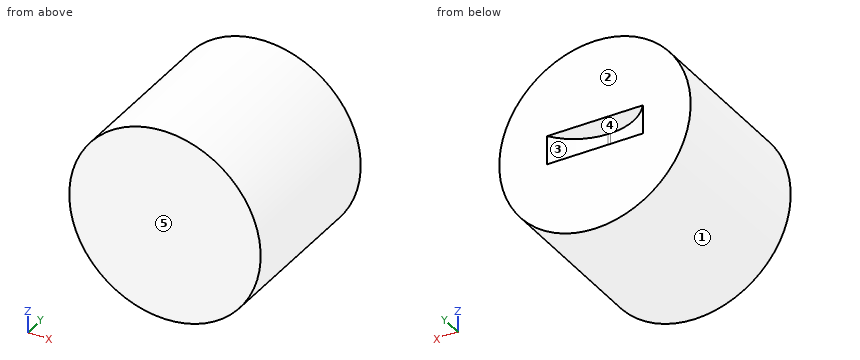
from build123d import *

# Parameters (mm, degrees)
SKETCH1_R           = 20
BOSS_EXTRUDE1_DEPTH = 35
SKETCH2_W           = 20
SKETCH2_H           = 6
CUT_EXTRUDE1_DEPTH  = 5
FILLET1_R           = 12


with BuildPart() as part:
    # Sketch1 → Boss-Extrude1 (new body)
    with BuildSketch(Plane(origin=(0, 0, 0), x_dir=(1, 0, 0), z_dir=(0, 1, 0))):
        with Locations(Location((0, 0, 0), (0, 0, 270))):
            Circle(SKETCH1_R)
    extrude(amount=BOSS_EXTRUDE1_DEPTH)

    # Sketch2 → Cut-Extrude1 (cut)
    with BuildSketch(Plane(origin=(0, 35, 0), x_dir=(1, 0, 0), z_dir=(0, 1, 0))):
        Rectangle(SKETCH2_W, SKETCH2_H)
    extrude(amount=-CUT_EXTRUDE1_DEPTH, mode=Mode.SUBTRACT)

    # Fillet1
    # the kernel refuses this fillet: 12 mm, written as the material it adds along each edge
    with BuildSketch(Plane(origin=(10, 30, 3), x_dir=(0, 1, 0), z_dir=(0, 0, -1)), Plane(origin=(-10, 30, -3), x_dir=(0, 1, 0), z_dir=(0, 0, 1))) as fillet1_piece_1:
        with BuildLine():
            CenterArc((12, -9.746794345), FILLET1_R, 125.685334713, 54.314665287)
            Line((0, -9.746794345), (0, 0))
            Line((0, 0), (5, 0))
        make_face()
    extrude(amount=6)


solid = part.part
Read the model definition and answer for the solid it produces. Units are mm, in the model's axes. Face numbers are marked on the shaded views. A direction names the side the tool comes from. Give positions to 0.01 mm unless a question says otherwise; leave off trailing zeros. Loops run counter-clockwise (first coordinate to the right, second up) from the corner with the lowest first, then second, coordinate; pieces in that order, holes last. Notation, with made-up numbers: (53, -24) - (95, -24) arc R20 cw to (95, 0) - close; hole circle Ø11 at (-40, 75.5). An arc over 180 degrees is marked (long way). Answer as CSV lines item,"result". Start each with the question number.
1) Find section A-A (z = 0). Write down the section's boundary in (x, y), then the cut area to 3 significant figures.
2) Each of these flat-tipped pins is pushed along its axis until it touches: pin 1 Ø2.5 at (x, y) = (4, 33) entering from -Z; pin 2 Ø6 at (y, z) = (16.5, 12) entering from -X; pin 3 Ø5 at (y, z) = (25, 14) entering from +X. Where does it stop, or does it pass through?
3) Determine the mould class of the marked faces 1, 2 and 3 for opening direction Z: released by +Z, released by -Z, zero draft, split by the parting line, or undercut.
4) Which of the six approach directions +Z, -Z, +X, -X, +Y, -Y give full straight-line access (tool end or side, diameter ignored) to the marked faces 4 and 5?
5) Straight lines are drawn through the part: L1, parallel to Z at x = 9.5, y = 16; L2, parallel to Z at x = -5, y = 15; L3, parallel to X at y = 25, z = 15. For each, find the intervals that lie inside material, in ascending order. Write a range as from..to.
6) Find section B-B (y = 27). Write down the section's boundary in (x, z), then the cut area to 3 significant figures.
7) Find section D-D (z = -4.5). Write down the section's boundary in (x, y), then the cut area to 3 significant figures.
8) Find section C-C (x = 17). Write down the section's boundary in (y, z), then the cut area to 3 significant figures.
Findings below:
1,outline,"(-20, 0) - (20, 0) - (20, 35) - (10, 35) arc R12 cw to (0.25, 30) - (-0.25, 30) arc R12 cw to (-10, 35) - (-20, 35) - close"
1,area,"1,330 mm^2"
2,pin 1,"z = -19.81"
2,pin 2,"x = -17.86"
2,pin 3,"x = 16.36"
3,face 1,"split by the parting line"
3,face 2,"zero draft"
3,face 3,"undercut"
4,face 4,"+Y"
4,face 5,"+Z, -Z, +X, -X, -Y"
5,L1,"-17.6..17.6"
5,L2,"-19.36..19.36"
5,L3,"-13.23..13.23"
6,outline,"circle Ø40 at (0, 0)"
6,area,"1,260 mm^2"
7,outline,"(-19.49, 0) - (19.49, 0) - (19.49, 35) - (-19.49, 35) - close"
7,area,"1,360 mm^2"
8,outline,"(0, -10.54) - (35, -10.54) - (35, 10.54) - (0, 10.54) - close"
8,area,"737 mm^2"
